The figure shows three views and two pictorial views of one solid part (mm, origin at its lowest corner). Answer the questions. A direction names the side the tool comes from. Round coordinates to 2 decimals unless told otherwise and drop trailing zeros. Loops run counter-clockwise (first coordinate to the right, second up) from the corner with the lowest first, then second, coordinate; pieces in that order, holes last. Notation, with made-up numbers: (46, 77.5) -> (62, 77.5) arc R23 cw to (62, 101.5) -> close; hole circle Ø9 at (-34.75, -14.75). An arc over 180 degrees is marked (long way). Put each result on its own line as item: value.
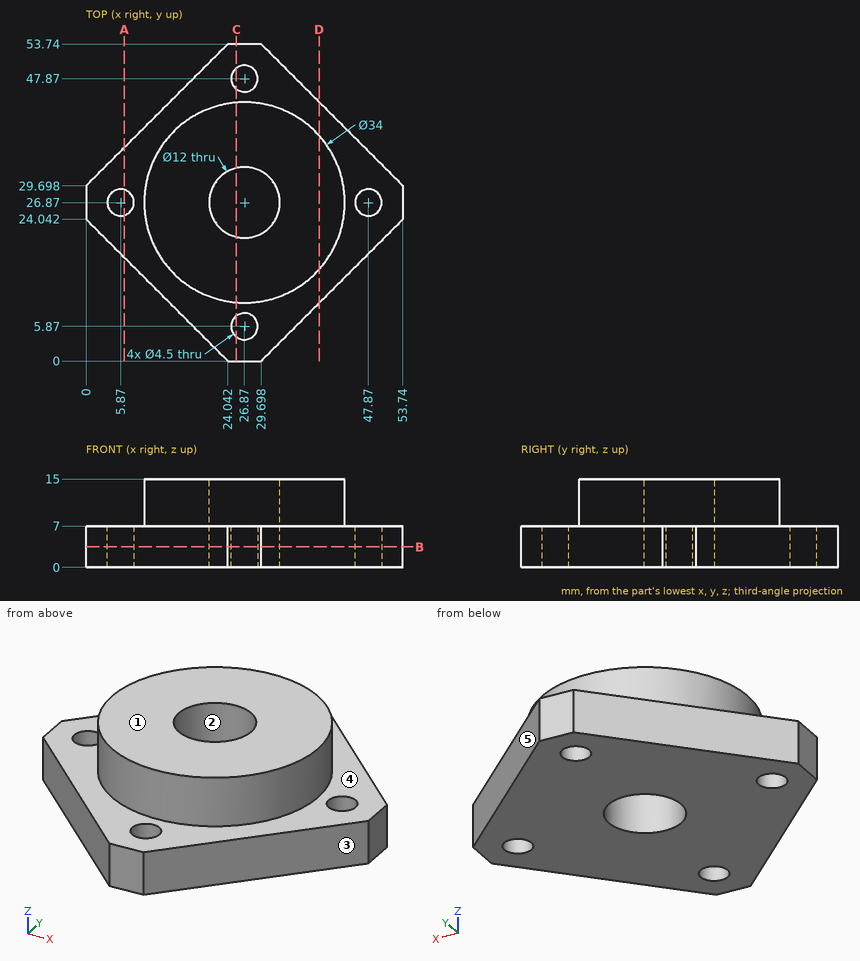
Item 1: The part is cut by section D-D (x = 39.5). Determine the outline of the cut face in (y, z).
Derived:
outline: (9.8, 0) -> (43.94, 0) -> (43.94, 7) -> (38.25, 7) -> (38.25, 15) -> (15.49, 15) -> (15.49, 7) -> (9.8, 7) -> close
Item 2: Flat-ended cylindrical pins translate along their axes: pin 1 Ø6 at (x, y) = (26.87, 5.87) entering from +Z; pin 2 Ø2 at (x, y) = (41, 27.5) entering from -Z; pin 3 Ø2 at (y, z) = (46, 7) entering from -X; pin 4 Ø6 at (y, z) = (10.5, 3) entering from -X. Find the tip coordinate at first contact, or state that the pin passes through.
Derived:
pin 1: stops at z = 7
pin 2: stops at z = 0
pin 3: stops at x = 15.3
pin 4: stops at x = 10.54
Item 3: The part is cut by section B-B (z = 3.5). Determine the outline of the cut face in (x, y), then the cut area to 3 significant figures.
Derived:
outline: (0, 24.04) -> (24.04, 0) -> (29.7, 0) -> (53.74, 24.04) -> (53.74, 29.7) -> (29.7, 53.74) -> (24.04, 53.74) -> (0, 29.7) -> close; hole circle Ø4.5 at (5.87, 26.87); hole circle Ø12 at (26.87, 26.87); hole circle Ø4.5 at (26.87, 5.87); hole circle Ø4.5 at (26.87, 47.87); hole circle Ø4.5 at (47.87, 26.87)
area: 1,560 mm^2
Item 4: Find the intervals of material crossed by line 1 along X through (y, z) = (27, 10.75); line 2 along X through (y, z) = (28, 3.75) (1 decimal); line 3 along Y through (x, z) = (28.5, 1) (1 decimal), in increasing order.
Derived:
line 1: x = 9.87 to 20.87, 32.87 to 43.87
line 2: x = 0 to 3.9, 7.8 to 21, 32.8 to 45.9, 49.8 to 53.7
line 3: y = 0 to 4.3, 7.4 to 21.1, 32.6 to 46.3, 49.4 to 53.7
Item 5: The part is cut by section A-A (x = 6.5). Determine the outline of the cut face in (y, z), then the cut area to 3 significant figures.
Derived:
outline: (17.54, 0) -> (24.71, 0) -> (24.71, 7) -> (17.54, 7) -> close; (29.03, 0) -> (36.2, 0) -> (36.2, 7) -> (29.03, 7) -> close
area: 100 mm^2
Item 6: The part is cut by section C-C (x = 25.5). Determine the outline of the cut face in (y, z) (1 decimal), then the cut area to 3 significant figures.
Derived:
outline: (0, 0) -> (4.1, 0) -> (4.1, 7) -> (0, 7) -> close; (7.7, 0) -> (21, 0) -> (21, 15) -> (9.9, 15) -> (9.9, 7) -> (7.7, 7) -> close; (32.7, 0) -> (46.1, 0) -> (46.1, 7) -> (43.8, 7) -> (43.8, 15) -> (32.7, 15) -> close; (49.7, 0) -> (53.7, 0) -> (53.7, 7) -> (49.7, 7) -> close
area: 422 mm^2
Item 7: For a pull along Y with two mould halves and no side action, classify the marked faces 1, 2 and 3 as pulls with the +Y half, pulls with the -Y half, needs draft (parallel to the pull), parting line crosses it, or undercut.
Derived:
face 1: needs draft
face 2: undercut
face 3: pulls with the -Y half
Item 8: Which of the six approach directions +Z, -Z, +X, -X, +Y, -Y give full straight-line access (tool end or side, diameter ignored) to the marked faces 4 and 5?
Derived:
face 4: +Z
face 5: +Z, -Z, +X, +Y
